```python
from build123d import *

# Parameters (mm, degrees)
F0_W     = 38.1
F0_H     = 38.1
F1_DEPTH = 38.1
F5_DEPTH = 38.1
F7_DEPTH = 38.1
F8_W     = 25.4
F8_H     = 7.62
F9_DEPTH = 38.1


with BuildPart() as f1:
    # F0 (on Front) → F1 (new body)
    with BuildSketch(Plane.XZ):
        with Locations((-19.05, 19.05)):
            Rectangle(F0_W, F0_H)
    extrude(amount=F1_DEPTH)

    # F4 (on offset) → F5 (cut)
    with BuildSketch(Plane.YZ):
        Polygon((-11.43, 15.875), (-6.35, 38.1), (-31.75, 38.1), (-26.67, 15.824118), (-21.59, 28.524118), (-16.51, 28.524118), align=None)
        Polygon((-38.1, 0), (-31.75, 0), (-38.1, 38.1), align=None)
        Polygon((-25.4, 0), (-12.7, 0), (-19.05, 15.875), align=None)
        Polygon((-6.35, 0), (0, 0), (0, 38.1), align=None)
    extrude(amount=-F5_DEPTH, mode=Mode.SUBTRACT)

    # F6 (on Front) → F7 (cut)
    with BuildSketch(Plane.XZ):
        Polygon((0, 0), (0, 38.1), (-6.35, 38.1), align=None)
        Polygon((-19.05, 22.225), (-12.7, 38.1), (-25.4, 38.1), align=None)
        Polygon((-38.1, 0), (-31.75, 38.1), (-38.1, 38.1), align=None)
        Polygon((-31.75, 0), (-6.35, 0), (-11.43, 22.225), (-16.51, 9.525), (-21.59, 9.525), (-26.67, 22.225), align=None)
    extrude(amount=F7_DEPTH, mode=Mode.SUBTRACT)

    # F8 (on offset) → F9 (cut)
    with BuildSketch(Plane.XY.offset(38.1)):
        with Locations((-25.4, -26.67)):
            Rectangle(F8_W, F8_H)
        with Locations((-12.7, -11.43)):
            Rectangle(F8_W, F8_H)
    extrude(amount=-F9_DEPTH, mode=Mode.SUBTRACT)


solid = f1.part
```
Input: part model. Units: mm. Frame: model coordinates. A direction names the side the tool comes from. Coordinates: 2 decimals unless noted, no trailing zeros. Order: outer loops, then holes, each group sorted by start corner. A loop starts at its lowest first (then second) coordinate and runs counter-clockwise, first axis right, second up. Notation, with made-up numbers: (-5.5, 78.25) - (50.5, 78.25) arc R6 cw to (50.5, 88.25) - close; hole circle Ø2 at (32, -4). An arc over 180 degrees is marked (long way). Return JSON: item names as keys, results as strings.
Q1. Cut plane D-D (z = 11). State how many separate pieces and enclosed holes the cut face has, then the cut area to 3 significant figures.
The answers:
{"separate pieces": "10", "enclosed holes": "0", "area": "309 mm2"}
Q2. Cut plane A-A (x = -22.5). Return loops of the section in (y, z) (3 decimals), then the cut area to 3 significant figures.
The answers:
{"outline": "(-36.892, 30.85) - (-33.717, 11.8) - (-30.48, 11.8) - (-30.48, 30.85) - close; (-22.86, 11.8) - (-20.68, 11.8) - (-19.05, 15.875) - (-17.42, 11.8) - (-15.24, 11.8) - (-15.24, 25.362) - (-16.51, 28.524) - (-21.59, 28.524) - (-22.86, 25.349) - close; (-7.62, 11.8) - (-4.383, 11.8) - (-1.208, 30.85) - (-7.62, 30.85) - close", "area": "301 mm2"}
Q3. Cut plane B-B (z = 26). Return loops of the section in (x, y), then the cut area to 3 significant figures.
The answers:
{"outline": "(-33.77, -36.08) - (-20.56, -36.08) - (-20.56, -30.48) - (-33.77, -30.48) - close; (-33.77, -22.6) - (-20.56, -22.6) - (-20.56, -15.5) - (-33.77, -15.5) - close; (-33.77, -9.12) - (-25.4, -9.12) - (-25.4, -7.62) - (-20.56, -7.62) - (-20.56, -2.02) - (-33.77, -2.02) - close; (-17.54, -36.08) - (-4.33, -36.08) - (-4.33, -28.99) - (-12.7, -28.99) - (-12.7, -30.48) - (-17.54, -30.48) - close; (-17.54, -22.6) - (-4.33, -22.6) - (-4.33, -15.5) - (-17.54, -15.5) - close; (-17.54, -7.62) - (-4.33, -7.62) - (-4.33, -2.02) - (-17.54, -2.02) - close", "area": "509 mm2"}
Q4. Draft query along X for faces 5 (the flat face through (-27, -19, 28.524)), 6 (the flat face through (-9.42, -5.65, 13.43)), 7 (the flat face through (-34.264, -33.39, 23.017)). Return one class per face: +X half, -X half, draft (parallel to the pull), parting line (faces both ways), or undercut.
The answers:
{"face 5": "draft", "face 6": "undercut", "face 7": "-X half"}
Q5. Ray query, probe 1 along X at (y, z) = (-5, 28.5); probe 2 along X at (y, z) = (-21, 12); probe 3 along Y at (x, z) = (-24, 16.5). Return the intervals inside material, ascending.
The answers:
{"probe 1": "x = -33.35 to -21.56, -16.54 to -4.75", "probe 2": "x = -36.1 to -29.01, -22.58 to -15.52, -9.09 to -2", "probe 3": "y = -34.5 to -30.48, -22.86 to -15.24, -7.62 to -3.6"}
Q6. First-contact query: pin 1 (7.5 mm diameter, centred on x = -27, z = 21.5, fed in from +Y); pin 2 (2 mm diameter, centred on y = -18, z = 22.5, fed in from -X); pin 3 (2.5 mm diameter, centred on x = -18, y = -6, fed in from -Z) (3 decimals); pin 4 (0.9 mm diameter, centred on y = -9.5, z = 29, fed in from +X). Flat tips, straight axial feed; report the tip coordinate or a pass-through.
The answers:
{"pin 1": "stops at y = -2.14", "pin 2": "stops at x = -34.52", "pin 3": "stops at z = 9.525", "pin 4": "passes through"}
Q7. Access query for faces 1 (the flat face through (-29.23, -8.926, 26.832)), 2 (the flat face through (-9.42, -25.21, 13.43)), 3 (the flat face through (-12.7, -30, 23)), 4 (the flat face through (-4.9, -22.2, 8)). Directions: +Z, -Z, +X, -X, +Y, -Y. A direction counts if a zero-diameter tool reaches every point of the face in a straight line with its end or side. Return the directions, or none.
The answers:
{"face 1": "+Z, +X, -X", "face 2": "-Z, +Y, -Y", "face 3": "+Z, -Z, -X", "face 4": "-Z, +X, -X"}
Q8. Cut plane C-C (z = 34.5). Return loops of the section in (x, y), then the cut area to 3 significant figures.
The answers:
{"outline": "(-32.35, -37.5) - (-23.96, -37.5) - (-23.96, -30.93) - (-32.35, -30.93) - close; (-32.35, -7.17) - (-23.96, -7.17) - (-23.96, -0.6) - (-32.35, -0.6) - close; (-14.14, -37.5) - (-5.75, -37.5) - (-5.75, -30.93) - (-14.14, -30.93) - close; (-14.14, -7.17) - (-5.75, -7.17) - (-5.75, -0.6) - (-14.14, -0.6) - close", "area": "221 mm2"}
